The model under review builds one solid part; all positions refer to its coordinate system, in mm. A direction names the side the tool comes from. Coordinates: 2 decimals unless noted, no trailing zeros. Order: outer loops, then holes, each group sorted by start corner. A loop starts at its lowest first (then second) coordinate and runs counter-clockwise, first axis right, second up. Notation, with made-up numbers: M -14,84 L 19,84 A20 ccw 19,116 Z; hole C 74.25,29 d3. An arc over 180 degrees is marked long. Write each question's results on one line, items separated by ' | '.
from build123d import *

# Parameters (mm, degrees)
SKETCH1_R           = 10
BOSS_EXTRUDE1_DEPTH = 9.3
SKETCH3_R           = 8
BOSS_EXTRUDE2_DEPTH = 1.8
SKETCH4_R           = 10
BOSS_EXTRUDE3_DEPTH = 93.9
SKETCH5_R           = 7.5
CUT_EXTRUDE1_DEPTH  = 5
SKETCH6_R           = 4.5
CUT_EXTRUDE2_DEPTH  = 95
SKETCH7_R           = 7.5
CUT_EXTRUDE3_DEPTH  = 5
CHAMFER1_SIZE       = 0.5


with BuildPart() as part:
    # Sketch1 → Boss-Extrude1 (new body)
    with BuildSketch(Plane.XY):
        Circle(SKETCH1_R)
    extrude(amount=BOSS_EXTRUDE1_DEPTH)

    # Sketch3 → Boss-Extrude2 (add)
    with BuildSketch(Plane.XY.offset(9.3)):
        Circle(SKETCH3_R)
    extrude(amount=BOSS_EXTRUDE2_DEPTH)

    # Sketch4 → Boss-Extrude3 (add)
    with BuildSketch(Plane.XY.offset(11.1)):
        Circle(SKETCH4_R)
    extrude(amount=BOSS_EXTRUDE3_DEPTH)

    # Sketch5 → Cut-Extrude1 (cut)
    with BuildSketch(Plane(origin=(0, 0, 0), x_dir=(-1, 0, 0), z_dir=(0, 0, -1))):
        Circle(SKETCH5_R)
    extrude(amount=-CUT_EXTRUDE1_DEPTH, mode=Mode.SUBTRACT)

    # Sketch6 → Cut-Extrude2 (cut)
    with BuildSketch(Plane(origin=(0, 0, 5), x_dir=(-1, 0, 0), z_dir=(0, 0, -1))):
        Circle(SKETCH6_R)
    extrude(amount=-CUT_EXTRUDE2_DEPTH, mode=Mode.SUBTRACT)

    # Sketch7 → Cut-Extrude3 (cut)
    with BuildSketch(Plane.XY.offset(105)):
        Circle(SKETCH7_R)
    extrude(amount=-CUT_EXTRUDE3_DEPTH, mode=Mode.SUBTRACT)

    # Chamfer1
    chamfer1_edges = [part.edges().sort_by_distance(p)[0] for p in [
        (-10, 0, 0),
        (-10, 0, 105),
    ]]
    chamfer(chamfer1_edges, length=CHAMFER1_SIZE)


solid = part.part
1) Take a section at A-A on y = 0. State the section outline as (x, z) points, plus the area to 3 significant figures.
Solutions:
outline: M -10,0.5 L -9.5,0 L -7.5,0 L -7.5,5 L -4.5,5 L -4.5,100 L -7.5,100 L -7.5,105 L -9.5,105 L -10,104.5 L -10,11.1 L -8,11.1 L -8,9.3 L -10,9.3 Z; M 4.5,5 L 7.5,5 L 7.5,0 L 9.5,0 L 10,0.5 L 10,9.3 L 8,9.3 L 8,11.1 L 10,11.1 L 10,104.5 L 9.5,105 L 7.5,105 L 7.5,100 L 4.5,100 Z | area: 1,090 mm2
2) To check wall thickness, follow line 1 along Z through (x, y) = (7.75, -3.5); line 2 along Y through (x, z) = (0, 3.1); line 3 along Y through (x, z) = (0, 76.5). State the ranges of each line that lie inside material, in increasing order.
Solutions:
line 1: 0 to 9.3, 11.1 to 105 | line 2: -10 to -7.5, 7.5 to 10 | line 3: -10 to -4.5, 4.5 to 10
3) Take a section at C-C on z = 41. State the section outline as (x, y) points.
Solutions:
outline: C 0,0 d20; hole C 0,0 d9
4) For faces 1 (the cylindrical face through (-7.493, 0.33, 102.535)), 2 (the flat face through (1, 8, 105)), 3 (the cylindrical face through (-2.17, -9.76, 57.15)), 4 (the cylindrical face through (7.493, 0.33, 2.465)), 5 (the flat face through (0, 8.2, 11.1)), list the 3-axis set-ups (+Z, -Z, +X, -X, +Y, -Y) from which the entire face can be reached by the end or side of a thin tool; tool diameter is ignored.
Solutions:
face 1: +Z | face 2: +Z, +X, -X, +Y, -Y | face 3: +Z, -Z | face 4: -Z | face 5: none
5) For pin 1 (1.5 mm diameter, centred on y = -5.5, z = 49.5, fed in from -X); pin 2 (12 mm diameter, centred on y = -4, z = 70, fed in from +X); pin 3 (7.5 mm diameter, centred on x = 1.5, y = -1.5, fed in from -Z); pin 4 (4.5 mm diameter, centred on x = -3.5, y = -2, fed in from +Z), all flat-tipped, find the tip position at first contact; note any pin that passes through.
Solutions:
pin 1: x = -8.8 | pin 2: x = 10 | pin 3: z = 5 | pin 4: z = 100
6) The part is to be moulded in two halves that separate along Y. For faces 6 (the flat face through (0, 8.2, 9.3)), 7 (the cylindrical face through (-1.73, -7.81, 10.19)), 8 (the flat face through (0, -5, 100)), say which applies: pulls with the +Y half, pulls with the -Y half, needs draft (parallel to the pull), parting line crosses it, or undercut.
Solutions:
face 6: needs draft | face 7: parting line crosses it | face 8: undercut
